Build history of the part. All positions in model axes, mm. A direction names the side the tool comes from. Round coordinates to 2 decimals unless told otherwise and drop trailing zeros. Write each loop counter-clockwise with the first axis right and the second up, starting at its lowest first coordinate (ties: lowest second). Pieces come first, ordered by that corner, then holes. Notation, with made-up numbers: (-34.5, 33.25) -> (-9.5, 33.25) arc R25 cw to (-9.5, 46.25) -> close; hole circle Ø9 at (78, 24.5). An arc over 180 degrees is marked (long way). Answer in a Markdown table with one row per item.
```python
from build123d import *

# Parameters (mm, degrees)
CORTE_EXTRUS_O1_DEPTH = 6
FILETE1_R             = 0.5


with BuildPart() as part:
    # Esboço1 → Revolução1 (revolve)
    with BuildSketch(Plane.XY):
        Polygon((0, -9.5), (0, 9.5), (-4, 9.5), (-4, 5.5), (-2, 5.5), (-2, -9.5), align=None)
    revolve(axis=Axis((0, -9.5, 0), (0, 1, 0)))

    # Esboço2 → Corte-extrusão1 (cut)
    with BuildSketch(Plane(origin=(0, 9.5, 0), x_dir=(1, 0, 0), z_dir=(0, 1, 0))):
        Polygon((1.5, -0.866025404), (1.5, 0.866025404), (0, 1.732050808), (-1.5, 0.866025404), (-1.5, -0.866025404), (0, -1.732050808), align=None)
    extrude(amount=-CORTE_EXTRUS_O1_DEPTH, mode=Mode.SUBTRACT)

    # Filete1
    filete1_edges = [part.edges().sort_by_distance(p)[0] for p in [
        (0.75, 3.5, 1.299038106),
        (-0.75, 3.5, 1.299038106),
        (-1.5, 3.5, 0),
        (-0.75, 3.5, -1.299038106),
        (0.75, 3.5, -1.299038106),
        (1.5, 3.5, 0),
        (2, -9.5, 0),
        (2, 5.5, 0),
        (4, 5.5, 0),
        (4, 9.5, 0),
    ]]
    fillet(filete1_edges, radius=FILETE1_R)


solid = part.part
```
Q1. Two-plate mould, pull along Z, no slides. Class faces 1 (the flat face through (2, 9.5, 0)), 2 (the flat face through (-1.5, 7, 0)), 3 (the cylindrical face through (0.867, 7.479, -3.905)), 4 (the cylindrical face through (-0.69, 3.65, -1.17)): released by +Z, released by -Z, zero draft, split by the parting line, or undercut.
A:
| item | result |
|---|---|
| face 1 | zero draft |
| face 2 | undercut |
| face 3 | split by the parting line |
| face 4 | undercut |
Q2. Saw through at D-D on y = 2.25. Write the cut outline in (x, z).
A:
| item | result |
|---|---|
| outline | circle Ø4 at (0, 0) |
Q3. Wall check: line 1 (Y direction, x = -2.75, z = -1.25); line 2 (Z direction, x = 0.75, y = 4.5); line 3 (X direction, y = 5, z = -1.25). Give the ranges that are in metal, low to high. Write a range as [from, to].
A:
| item | result |
|---|---|
| line 1 | [5.5, 9.5] |
| line 2 | [-1.85, -1.3], [1.3, 1.85] |
| line 3 | [-1.56, -0.83], [0.83, 1.56] |
Q4. Saw through at C-C on y = 4.25. Write the cut outline in (x, z), plus the area to 3 significant figures.
A:
| item | result |
|---|---|
| outline | circle Ø4 at (0, 0); hole (-1.5, -0.87) -> (0, -1.73) -> (1.5, -0.87) -> (1.5, 0.87) -> (0, 1.73) -> (-1.5, 0.87) -> close |
| area | 4.77 mm² |
Q5. Saw through at B-B on z = 0. Write the cut outline in (x, y).
A:
| item | result |
|---|---|
| outline | (-4, 6) arc R0.5 ccw to (-3.5, 5.5) -> (-2.5, 5.5) arc R0.5 cw to (-2, 5) -> (-2, -9) arc R0.5 ccw to (-1.5, -9.5) -> (1.5, -9.5) arc R0.5 ccw to (2, -9) -> (2, 5) arc R0.5 cw to (2.5, 5.5) -> (3.5, 5.5) arc R0.5 ccw to (4, 6) -> (4, 9) arc R0.5 ccw to (3.5, 9.5) -> (1.5, 9.5) -> (1.5, 4) arc R0.5 cw to (1, 3.5) -> (-1, 3.5) arc R0.5 cw to (-1.5, 4) -> (-1.5, 9.5) -> (-3.5, 9.5) arc R0.5 ccw to (-4, 9) -> close |
Q6. Drop flat-ended pins along their axis: P1, Ø2, axis at y = -1.5, z = 1, coming from the -X side; P2, Ø2, axis at y = -6.5, z = 0, coming from the +X side; P3, Ø2, axis at x = 0.5, z = -1.5, coming from the -Y side; P4, Ø1.5, axis at x = 2, y = -5.5, coming from the +Z side. Give the stop position or say it passes through.
A:
| item | result |
|---|---|
| P1 | x = -2 |
| P2 | x = 2 |
| P3 | y = -9.5 |
| P4 | z = 1.56 |
Q7. Which spindle directions (+Z, -Z, +X, -X, +Y, -Y) get a long thin tool onto all of the face, cutting with end or side? Do faces 5 (the cylindrical face through (0, -2, -2)), 6 (the flat face through (0, -9.5, 0)), 7 (the flat face through (-0.74, 6.788, -1.305)). Say none if no direction does.
A:
| item | result |
|---|---|
| face 5 | -Y |
| face 6 | +Z, -Z, +X, -X, -Y |
| face 7 | +Y |
Q8. Saw through at A-A on y = 7.25. Write the cut outline in (x, z), plus the area to 3 significant figures.
A:
| item | result |
|---|---|
| outline | circle Ø8 at (0, 0); hole (-1.5, -0.87) -> (0, -1.73) -> (1.5, -0.87) -> (1.5, 0.87) -> (0, 1.73) -> (-1.5, 0.87) -> close |
| area | 42.5 mm² |
